Autodesk Inventor part; units mm, degrees
ref_plane "YZ Plane" through (0, 0, 0) normal (1, 0, 0) x (0, 1, 0)
ref_plane "XZ Plane" through (0, 0, 0) normal (0, 1, 0) x (-1, 0, 0)
ref_plane "XY Plane" through (0, 0, 0) normal (0, 0, 1) x (1, 0, 0)
sketch "Sketch3" plane through (0, 0, 0) normal (0, 0, 1) x (1, 0, 0)
  line L0 (-311.15, 0) -> (0, 0)
  line L1 (0, 0) -> (-220.0163, 220.0163)
  line L2 (-301.625, 0) -> (-301.625, 38.1)
  line L3 (-301.625, 38.1) -> (-38.1, 38.1)
  line L4 (-23.0461, 23.0461) -> (-23.0461, 0)
  circle A0 centre (0, 0) radius 311.15
  point P0 (0, 0)
  point P1 (-306.9751, 50.8)
  dimension "d10" = 38.1
  dimension "d12" = 9.525
extrude "Extrusion3" add sketch "Sketch3" along normal blind 3.175 contours A0 L1 L3 L2 L0
sketch "Sketch4" plane through (0, 0, 0) normal (0, 0, -1) x (-1, 0, 0)
  line L0 (-141.2846, 157.1654) -> (-0.3893, 16.2701)
  line L1 (-145.7747, 152.6753) -> (-141.2846, 157.1654)
  line L2 (-4.8794, 11.78) -> (-145.7747, 152.6753)
  arc A0 (0, 0) -> (-4.8794, 11.78) centre (-16.6594, 0) ccw
  line L3 (0, -6.35) -> (0, 0)
  line L4 (6.35, -6.35) -> (0, -6.35)
  line L5 (6.35, -2.6303) -> (6.35, -6.35)
  arc A1 (5.6464, 5.6464) -> (-0.3893, 16.2701) centre (-16.6594, 0) ccw
  line L6 (6.35, -2.6303) -> (214.3556, 205.3753)
  line L7 (209.9135, 209.9135) -> (5.6464, 5.6464)
  arc A2 (214.3556, 205.3753) -> (209.9135, 209.9135) centre (0, 0) ccw
  circle A3 centre (245.7763, 172.0944) radius 1.5875
  circle A4 centre (271.9263, 126.8013) radius 1.5875
  circle A5 centre (289.814, 77.6554) radius 1.5875
  circle A6 centre (298.8958, 26.15) radius 1.5875
  circle A7 centre (304.7338, 6.35) radius 1.5875
  circle A8 centre (249.6775, 174.8261) radius 1.5875
  circle A9 centre (276.2426, 128.814) radius 1.5875
  circle A10 centre (294.4142, 78.888) radius 1.5875
  circle A11 centre (303.6401, 26.5651) radius 1.5875
  circle A12 centre (300.1694, 52.928) radius 1.5875
  circle A13 centre (286.4183, 104.2477) radius 1.5875
  circle A14 centre (263.9645, 152.4) radius 1.5875
  circle A15 centre (233.4903, 195.9217) radius 1.5875
  circle A16 centre (219.9695, 210.9892) radius 1.5875
  circle A17 centre (295.4793, 52.101) radius 1.5875
  circle A18 centre (281.943, 102.6189) radius 1.5875
  circle A19 centre (259.8401, 150.0188) radius 1.5875
  circle A20 centre (229.8421, 192.8604) radius 1.5875
  arc A21 (311.15, 0) -> (220.0163, 220.0163) centre (0, 0) ccw
  line L8 (220.0163, 220.0163) -> (0, 0)
  line L9 (0, 0) -> (311.15, 0)
  point P0 (-16.6594, 0)
  point P1 (-16.6594, 0)
  point P2 (0, 0)
extrude "Extrusion5" cut sketch "Sketch4" against normal through all contours A3 | A4 | A5 | A7 | A8 | A9 | A10 | A12 | A13 | A14 | A15 | A16 | A17 | A18 | A19 | A20
properties part number "Side Panel 2" material "Polycarbonate, Clear"
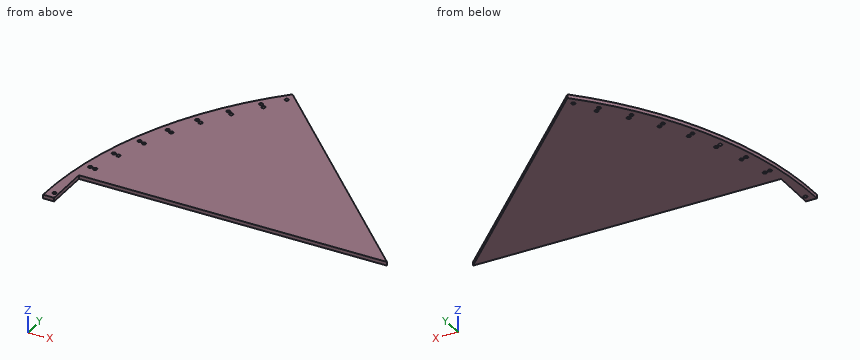
Work out the finished part from the listing and answer in its coordinate system (mm). Round coordinates to 2 decimals unless told otherwise and drop trailing zeros. Write each loop counter-clockwise with the first axis right and the second up, starting at its lowest first coordinate (ties: lowest second). Pieces come first, ordered by that corner, then holes.
1) A cutting plane is placed at B-B on x = -78. Determine the outline of the cut face in (y, z) (3 decimals).
2) A cutting plane is placed at C-C on x = -144.5. Determine the outline of the cut face in (y, z) (3 decimals).
3) Consider probe 1 along X at (y, z) = (171, 2.15); probe 2 along Y at (x, z) = (-50.5, 2.75); probe 3 along Y at (x, z) = (-243, 2.6). Determine where each line is inside the solid, lowest interval first.
4) A cutting plane is placed at A-A on z = 1.95. Give the number of separate pieces and of enclosed holes in the cut face, and give its area (3 significant figures).
5) Flat-ended cylindrical pins translate along their axes: P1, Ø1.9, axis at x = -289.81, y = 77.66, coming from the +Z side; P2, Ø1, axis at y = 19, z = 2, coming from the +X side (3 decimals); P3, Ø1.5, axis at x = -140.5, z = 1, coming from the +Y side. Find the tip coordinate at first contact, or state that the pin passes through.
Entries:
1. outline: (38.1, 0) - (78, 0) - (78, 3.175) - (38.1, 3.175) - close
2. outline: (38.1, 0) - (144.5, 0) - (144.5, 3.175) - (38.1, 3.175) - close
3. probe 1: x = -259.95 to -246.93, -244.63 to -171
3. probe 2: y = 38.1 to 50.5
3. probe 3: y = 38.1 to 194.33
4. separate pieces: 1
4. enclosed holes: 16
4. area: 27,100 mm2
5. P1: passes through
5. P2: stops at x = -301.625
5. P3: stops at y = 141.25
